Design review of the part built by this model. Coordinates are the model's own, in mm. Face numbers are marked on the shaded views. A direction names the side the tool comes from. Coordinates: 2 decimals unless noted, no trailing zeros. Loops run counter-clockwise (first coordinate to the right, second up) from the corner with the lowest first, then second, coordinate; pieces in that order, holes last. Notation, with made-up numbers: (58, 48) - (112, 48) arc R6 ccw to (112, 59) - close; hole circle Ø7 at (70, 69). An arc over 180 degrees is marked (long way). One line per question, with ' | ' between items.
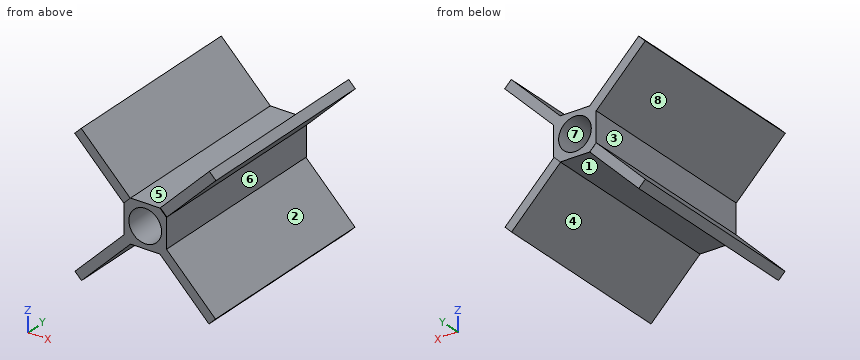
from build123d import *

# Parameters (mm, degrees)
SKETCH1_W           = 13
SKETCH1_H           = 13
BOSS_EXTRUDE1_DEPTH = 59.5
CHAMFER1_SIZE       = 2
SKETCH6_W           = 2.828427124
SKETCH6_H           = 59.370634799
BOSS_EXTRUDE3_DEPTH = 21.22
SKETCH5_W           = 2.828427124
SKETCH5_H           = 59.460523053
BOSS_EXTRUDE2_DEPTH = 21.22
SKETCH7_W           = 2.828427124
SKETCH7_H           = 59.614279407
BOSS_EXTRUDE4_DEPTH = 21.22
SKETCH8_W           = 2.828427124
SKETCH8_H           = 59.32576951
BOSS_EXTRUDE5_DEPTH = 21.22
SKETCH10_R          = 5
CUT_EXTRUDE2_DEPTH  = 67.923655478


with BuildPart() as part:
    # Sketch1 → Boss-Extrude1 (new body)
    with BuildSketch(Plane(origin=(0, 0, 0), x_dir=(1, 0, 0), z_dir=(0, 1, 0))):
        Rectangle(SKETCH1_W, SKETCH1_H)
    extrude(amount=BOSS_EXTRUDE1_DEPTH)

    # Chamfer1
    chamfer1_edges = [part.edges().sort_by_distance(p)[0] for p in [
        (6.5, 29.75, 6.5),
        (-6.5, 29.75, 6.5),
        (-6.5, 29.75, -6.5),
        (6.5, 29.75, -6.5),
    ]]
    chamfer(chamfer1_edges, length=CHAMFER1_SIZE)

    # Sketch6 → Boss-Extrude3 (add)
    with BuildSketch(Plane(origin=(5.5, 0, -5.5), x_dir=(-0.7071067811865465, 0, -0.7071067811865487), z_dir=(0.7071067811865487, 0, -0.7071067811865465))):
        with Locations((0, 29.6853174)):
            Rectangle(SKETCH6_W, SKETCH6_H)
    extrude(amount=BOSS_EXTRUDE3_DEPTH)

    # Sketch5 → Boss-Extrude2 (add)
    with BuildSketch(Plane(origin=(-5.5, 0, -5.5), x_dir=(-0.7071067811865487, 0, 0.7071067811865465), z_dir=(-0.7071067811865465, 0, -0.7071067811865487))):
        with Locations((0, 29.730261527)):
            Rectangle(SKETCH5_W, SKETCH5_H)
    extrude(amount=BOSS_EXTRUDE2_DEPTH)

    # Sketch7 → Boss-Extrude4 (add)
    with BuildSketch(Plane(origin=(-5.5, 0, 5.5), x_dir=(0.7071067811865465, 0, 0.7071067811865487), z_dir=(-0.7071067811865487, 0, 0.7071067811865465))):
        with Locations((0, 29.692860297)):
            Rectangle(SKETCH7_W, SKETCH7_H)
    extrude(amount=BOSS_EXTRUDE4_DEPTH)

    # Sketch8 → Boss-Extrude5 (add)
    with BuildSketch(Plane(origin=(5.5, 0, 5.5), x_dir=(0.7071067811865487, 0, -0.7071067811865465), z_dir=(0.7071067811865465, 0, 0.7071067811865487))):
        with Locations((0, 29.837115245)):
            Rectangle(SKETCH8_W, SKETCH8_H)
    extrude(amount=BOSS_EXTRUDE5_DEPTH)

    # Sketch10 → Cut-Extrude2 (cut, through all)
    with BuildSketch(Plane(origin=(0, 59.5, 0), x_dir=(1, 0, 0), z_dir=(0, 1, 0))):
        with Locations(Location((0, 0, 0), (0, 0, 270))):
            Circle(SKETCH10_R)
    extrude(amount=-CUT_EXTRUDE2_DEPTH, mode=Mode.SUBTRACT)


solid = part.part
Q1. To check wall thickness, follow line 1 along X through (y, z) = (30, 0); line 2 along Y through (x, z) = (-8.5, -8); line 3 along X through (y, z) = (37.5, -2.5). State the ranges of each line that lie inside material, in increasing order.
Returned:
line 1: x = -6.5 to -5, 5 to 6.5 | line 2: y = 0 to 59.46 | line 3: x = -6.5 to -4.33, 4.33 to 6.5
Q2. Take a section at A-A (x = 0). Give the boundary of the cut face in (y, z).
Returned:
outline: (0, -6.5) - (59.5, -6.5) - (59.5, -5) - (0, -5) - close; (0, 5) - (59.5, 5) - (59.5, 6.5) - (0, 6.5) - close
Q3. Draft analysis for pull direction X (two halves, no side actions). For the marked faces 1, 2 and 3, state which applies: +X half, -X half, draft (parallel to the pull), parting line (faces both ways), or undercut.
Returned:
face 1: undercut | face 2: +X half | face 3: -X half
Q4. Take a section at B-B (z = 0). Give the boundary of the cut face in (x, y).
Returned:
outline: (-6.5, 0) - (-5, 0) - (-5, 59.5) - (-6.5, 59.5) - close; (5, 0) - (6.5, 0) - (6.5, 59.5) - (5, 59.5) - close
Q5. For pin 1 (6 mm diameter, centred on x = 6.5, y = 12.5, fed in from +Z); pin 2 (13.5 mm diameter, centred on x = 14, z = -16, fed in from +Y); pin 3 (8.5 mm diameter, centred on x = -15, z = -13, fed in from +Y), all flat-tipped, find the tip position at first contact; note any pin that passes through.
Returned:
pin 1: stops at z = 11.5 | pin 2: stops at y = 59.37 | pin 3: stops at y = 59.46
Q6. Tool access review of the marked faces 4, 5, 6, 7 and 8: name each direction out of +Z, -Z, +X, -X, +Y, -Y from which nothing blocks a thin tool from reaching the whole face with its end or side.
Returned:
face 4: -Z, +Y, -Y | face 5: +Z, +Y, -Y | face 6: +X, +Y, -Y | face 7: +Y, -Y | face 8: -X, +Y, -Y
Q7. Take a section at C-C (y = 19.5). Give the boundary of the cut face in (x, z).
Returned:
outline: (-21.5, -19.5) - (-19.5, -21.5) - (-4.5, -6.5) - (4.5, -6.5) - (19.5, -21.5) - (21.5, -19.5) - (6.5, -4.5) - (6.5, 4.5) - (21.5, 19.5) - (19.5, 21.5) - (4.5, 6.5) - (-4.5, 6.5) - (-19.5, 21.5) - (-21.5, 19.5) - (-6.5, 4.5) - (-6.5, -4.5) - close; hole circle Ø10 at (0, 0)
